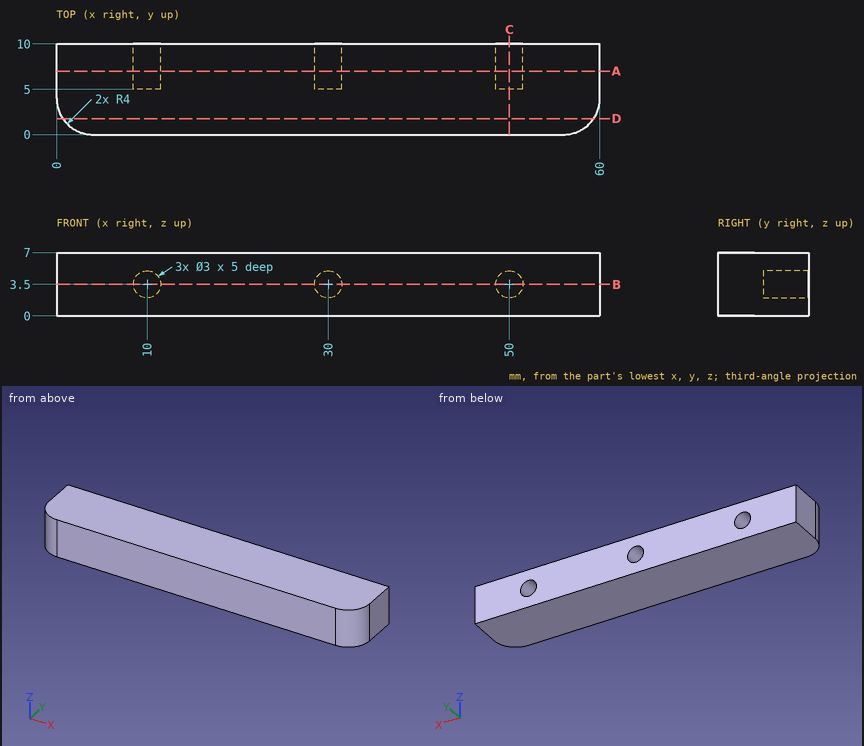
Check sheet for the drawn part. Datum: minimum x, y, z corner. Units: mm. Round coordinates to 2 decimals unless told otherwise and drop trailing zeros. Order: outer loops, then holes, each group sorted by start corner. A loop starts at its lowest first (then second) coordinate and runs counter-clockwise, first axis right, second up.
1) Section check A-A (y = 7). Record the boundary of the cut face in (x, z).
2) Go/stop test with flat-tipped pins: pin 1 Ø4 at (y, z) = (8, 3.5) entering from -X; pin 2 Ø0.9 at (x, z) = (50, 4) entering from +Y. Record where each tip stops, or that it passes through.
3) Section check C-C (x = 50). Record the boundary of the cut face in (y, z), and give its area (3 significant figures).
4) Section check D-D (y = 1.75). Record the boundary of the cut face in (x, z).
5) Section check B-B (z = 3.5). Record the boundary of the cut face in (x, y).
6) Scan lines: line 1 (X direction, y = 8.4, z = 3.5); line 2 (Y direction, x = 30, z = 4.25); line 3 (Z direction, x = 50.5, y = 7). Record each from-to range of solid material in increasing order.
Result:
1. outline: (0, 0) - (60, 0) - (60, 7) - (0, 7) - close; hole circle Ø3 at (10, 3.5); hole circle Ø3 at (30, 3.5); hole circle Ø3 at (50, 3.5)
2. pin 1: stops at x = 0
2. pin 2: stops at y = 5
3. outline: (0, 0) - (10, 0) - (10, 2) - (5, 2) - (5, 5) - (10, 5) - (10, 7) - (0, 7) - close
3. area: 55.0 mm2
4. outline: (0.69, 0) - (59.31, 0) - (59.31, 7) - (0.69, 7) - close
5. outline: (0, 4) arc R4 ccw to (4, 0) - (56, 0) arc R4 ccw to (60, 4) - (60, 10) - (51.5, 10) - (51.5, 5) - (48.5, 5) - (48.5, 10) - (31.5, 10) - (31.5, 5) - (28.5, 5) - (28.5, 10) - (11.5, 10) - (11.5, 5) - (8.5, 5) - (8.5, 10) - (0, 10) - close
6. line 1: x = 0 to 8.5, 11.5 to 28.5, 31.5 to 48.5, 51.5 to 60
6. line 2: y = 0 to 5
6. line 3: z = 0 to 2.09, 4.91 to 7
